Check sheet for the modelled part. Datum: model origin and axes. Units: mm. A direction names the side the tool comes from. Give positions to 0.01 mm unless a question says otherwise; leave off trailing zeros. Loops run counter-clockwise (first coordinate to the right, second up) from the corner with the lowest first, then second, coordinate; pieces in that order, holes last. Notation, with made-up numbers: (10, -22) -> (51, -22) arc R7 ccw to (51, -11) -> close; hole circle Ø1 at (-1.75, 79.5). An arc over 180 degrees is marked (long way). Write each question's results on one line, items separated by ' | '. Start each with the question number.
1. Material ranges on L1, parallel to Y at x = 36.25, z = 1.5; L2, parallel to Y at x = 40, z = 18; L3, parallel to Y at x = 39.75, z = 10.25, recorded low to high. Write a range as from..to.
2. Gauge pin test, flat ends, axial feed: pin 1 Ø1.3 at (x, z) = (35, 8.5) entering from -Y; pin 2 Ø3.5 at (x, y) = (37, 81.5) entering from -Z; pin 3 Ø4 at (x, z) = (37, -3.5) entering from -Y. Record the tip position at first contact, or that the pin passes through.
3. Cross-section at D-D on z = 2. Record the boundary of the cut face in (x, y), and give its area (3 significant figures).
4. Mould release check, pull along X, two halves, no side actions. Record for faces 6 (the face through (41.206, 84.851, 2.465)), 7 (the face through (36.61, 41.09, 11.33)), 8 (the face through (41, 71, 23)), 9 (the face through (40.11, 41.07, 11.34)): +X half, -X half, draft (parallel to the pull), parting line (faces both ways), or undercut.
5. Cross-section at C-C on z = 12.75. Record the boundary of the cut face in (x, y), and give its area (3 significant figures).
6. Cross-section at B-B on y = 93. Record the boundary of the cut face in (x, z).
7. Tool access check on faces 1 (the face through (42, 42.58, 11)), 2 (the face through (38, 57, -7)), 3 (the face through (35, 42.58, 11)), 4 (the face through (38, 86, 5)), 5 (the face through (34.271, 70.581, 21.496)). Record the directions out of +Z, -Z, +X, -X, +Y, -Y that give a thin tool (end or side, any length) a straight path to the whole face; none if there is none.
8. Cross-section at A-A on x = 36.75. Record the boundary of the cut face in (y, z), and give its area (3 significant figures).
Autodesk Fusion 360 part; units mm, degrees
sketch "Poarta Dreapta Sus" plane through (0, 0, 0) normal (0, 0, 1) x (1, 0, 0)
  line L0 (39.3447, 42.5803) -> (39.3447, 41.5803)
  line L1 (40.8447, 40.5803) -> (39.3447, 41.5803)
  line L2 (40.8447, 40.5803) -> (35.8447, 40.5803)
  line L3 (37.3447, 41.5803) -> (35.8447, 40.5803)
  line L4 (37.3447, 42.5803) -> (37.3447, 41.5803)
  circle A0 centre (38.3447, 56.5803) radius 3
  circle A1 centre (38.3447, 56.5803) radius 5.5
  circle A2 centre (38.3447, 85.7526) radius 5.5
  circle A3 centre (38.3447, 85.7526) radius 3
  line L5 (43.8447, 99.7526) -> (32.8447, 99.7526)
  line L6 (43.8447, 99.7526) -> (43.8447, 42.5803)
  line L7 (32.8447, 99.7526) -> (32.8447, 42.5803)
  line L8 (43.8447, 42.5803) -> (32.8447, 42.5803)
  line L9 (39.3447, 99.7526) -> (39.3447, 98.7526)
  line L10 (37.3447, 99.7526) -> (37.3447, 98.7526)
  line L11 (40.8447, 97.7526) -> (35.8447, 97.7526)
  line L12 (38.3447, 99.7526) -> (38.3447, 97.7526) construction
  line L13 (39.3447, 98.7526) -> (40.8447, 97.7526)
  line L14 (37.3447, 98.7526) -> (35.8447, 97.7526)
  point P0 (38.3447, 99.7526)
  dimension "d718" = 1
  dimension "d719" = 1
  dimension "d720" = 2
  dimension "d721" = 2.5
  dimension "d722" = 6
  dimension "d723" = 57.1723
  dimension "d724" = 5
  dimension "d725" = 32.8447
  dimension "d726" = 42.5803
  dimension "d727" = 2
  dimension "d728" = 3
  dimension "d729" = 14
  dimension "d730" = 43.1723
  dimension "d731" = 1
  dimension "d732" = 1
  dimension "d733" = 5
  dimension "d734" = 2
extrude "Extrude1" add sketch "Poarta Dreapta Sus" along normal blind 23 contours A1 L6 L7 L8 | L0 L1 L2 L3 L4 L8 | A1 | A1 A2 L6 L7 | A2 | A2 L5 L6 L7 L9 L10 L11 L13 L14
extrude "Extrude2" add sketch "Poarta Dreapta Sus" along normal blind 18 from surface at 5 contours A3
extrude "Extrude3" add sketch "Poarta Dreapta Sus" along normal blind 23 contours A0
extrude "Extrude4" add sketch "Poarta Dreapta Sus" against normal blind 7 contours A0
fillet "Fillet1" radius 5 2 edges at (32.8447, 71.1664, 23) (32.8447, 71.1664, 23)
Geometry says:
1) L1: 40.58..40.85, 42.58..83.6, 87.9..97.75, 98.02..99.75 | L2: 40.58..41.14, 42.58..97.75, 98.32..99.75 | L3: 40.58..41.31, 42.58..97.75, 98.48..99.75
2) pin 1: y = 42.58 | pin 2: z = 0 | pin 3: y = 53.58
3) outline: (32.84, 42.58) -> (37.34, 42.58) -> (37.34, 41.58) -> (35.84, 40.58) -> (40.84, 40.58) -> (39.34, 41.58) -> (39.34, 42.58) -> (43.84, 42.58) -> (43.84, 99.75) -> (39.34, 99.75) -> (39.34, 98.75) -> (40.84, 97.75) -> (35.84, 97.75) -> (37.34, 98.75) -> (37.34, 99.75) -> (32.84, 99.75) -> close; hole circle Ø6 at (38.34, 85.75) | area: 601 mm^2
4) face 6: undercut | face 7: -X half | face 8: draft | face 9: +X half
5) outline: (32.84, 42.58) -> (37.34, 42.58) -> (37.34, 41.58) -> (35.84, 40.58) -> (40.84, 40.58) -> (39.34, 41.58) -> (39.34, 42.58) -> (43.84, 42.58) -> (43.84, 99.75) -> (39.34, 99.75) -> (39.34, 98.75) -> (40.84, 97.75) -> (35.84, 97.75) -> (37.34, 98.75) -> (37.34, 99.75) -> (32.84, 99.75) -> close | area: 629 mm^2
6) outline: (32.84, 0) -> (43.84, 0) -> (43.84, 23) -> (37.84, 23) arc R5 ccw to (32.84, 18) -> close
7) face 1: +Z, -Z, +X | face 2: -Z, +X, -X, +Y, -Y | face 3: +Z, -Z, -X | face 4: -Z | face 5: +Z, -X, +Y, -Y
8) outline: (40.58, 0) -> (41.18, 0) -> (41.18, 22.88) -> (40.58, 22.88) -> close; (42.58, 0) -> (54.04, 0) -> (54.04, -7) -> (59.12, -7) -> (59.12, 0) -> (83.21, 0) -> (83.21, 5) -> (88.29, 5) -> (88.29, 0) -> (97.75, 0) -> (97.75, 22.88) -> (42.58, 22.88) -> close; (98.36, 0) -> (99.75, 0) -> (99.75, 22.88) -> (98.36, 22.88) -> close | area: 1,320 mm^2
